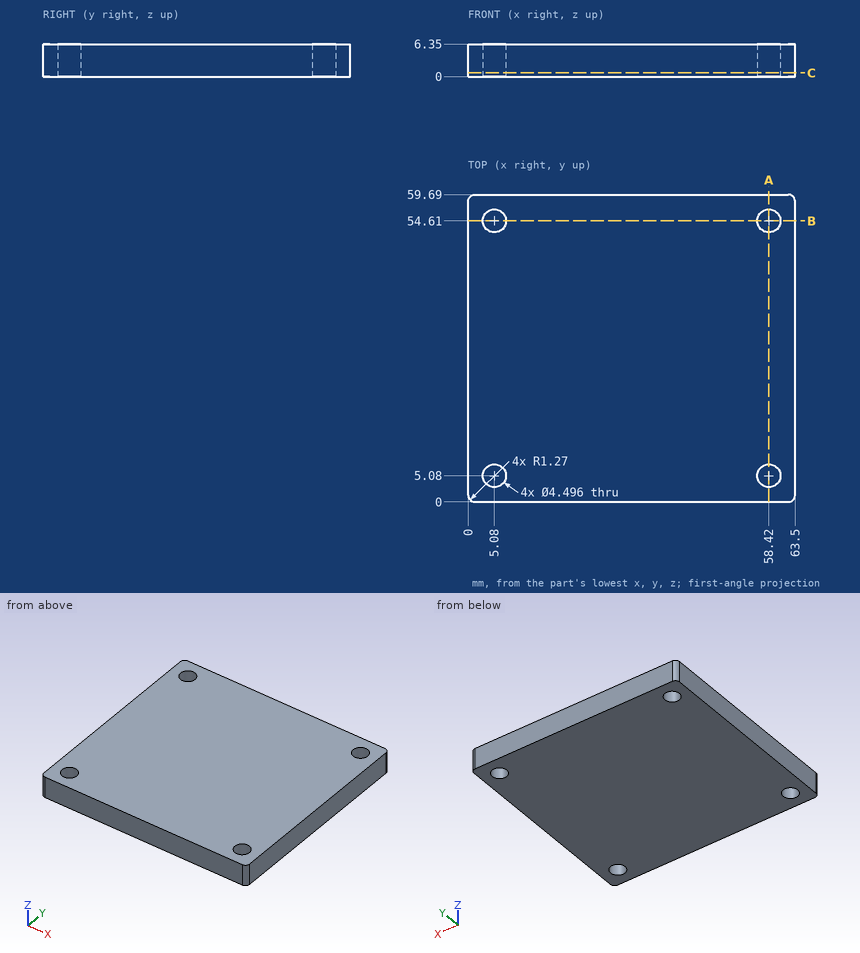
The figure shows three views and two pictorial views of one solid part (mm, origin at its lowest corner). Answer the questions. Round coordinates to 2 decimals unless told otherwise and drop trailing zeros. Write each loop counter-clockwise with the first axis right and the second up, starting at its lowest first coordinate (ties: lowest second). Pieces come first, ordered by that corner, then holes. Notation, with made-up numbers: M 88.25,-20 L 101.25,-20 A37 ccw 101.25,17 Z; hole C 86.25,-11 d4. An arc over 180 degrees is marked long. Write each question's results on one line, items separated by ' | '. Start each with the question number.
(1) The part is cut by section B-B, the plane y = 54.61. Write down the section's boundary in (x, z).
(2) Find the intervals of material crossed by line 1 (Y direction, x = 58.42, z = 3); line 2 (Y direction, x = 57.5, z = 1.5); line 3 (X direction, y = 4, z = 4.5), in increasing order.
(3) The part is cut by section A-A, the plane x = 58.42. Write down the section's boundary in (y, z).
(4) The part is cut by section C-C, the plane z = 0.75. Write down the section's boundary in (x, y).
Worked answers:
1) outline: M 0,0 L 2.83,0 L 2.83,6.35 L 0,6.35 Z; M 7.33,0 L 56.17,0 L 56.17,6.35 L 7.33,6.35 Z; M 60.67,0 L 63.5,0 L 63.5,6.35 L 60.67,6.35 Z
2) line 1: y = 0 to 2.83, 7.33 to 52.36, 56.86 to 59.69 | line 2: y = 0 to 3.03, 7.13 to 52.56, 56.66 to 59.69 | line 3: x = 0 to 3.11, 7.05 to 56.45, 60.39 to 63.5
3) outline: M 0,0 L 2.83,0 L 2.83,6.35 L 0,6.35 Z; M 7.33,0 L 52.36,0 L 52.36,6.35 L 7.33,6.35 Z; M 56.86,0 L 59.69,0 L 59.69,6.35 L 56.86,6.35 Z
4) outline: M 0,1.27 A1.27 ccw 1.27,0 L 62.23,0 A1.27 ccw 63.5,1.27 L 63.5,58.42 A1.27 ccw 62.23,59.69 L 1.27,59.69 A1.27 ccw 0,58.42 Z; hole C 5.08,5.08 d4.5; hole C 5.08,54.61 d4.5; hole C 58.42,5.08 d4.5; hole C 58.42,54.61 d4.5
